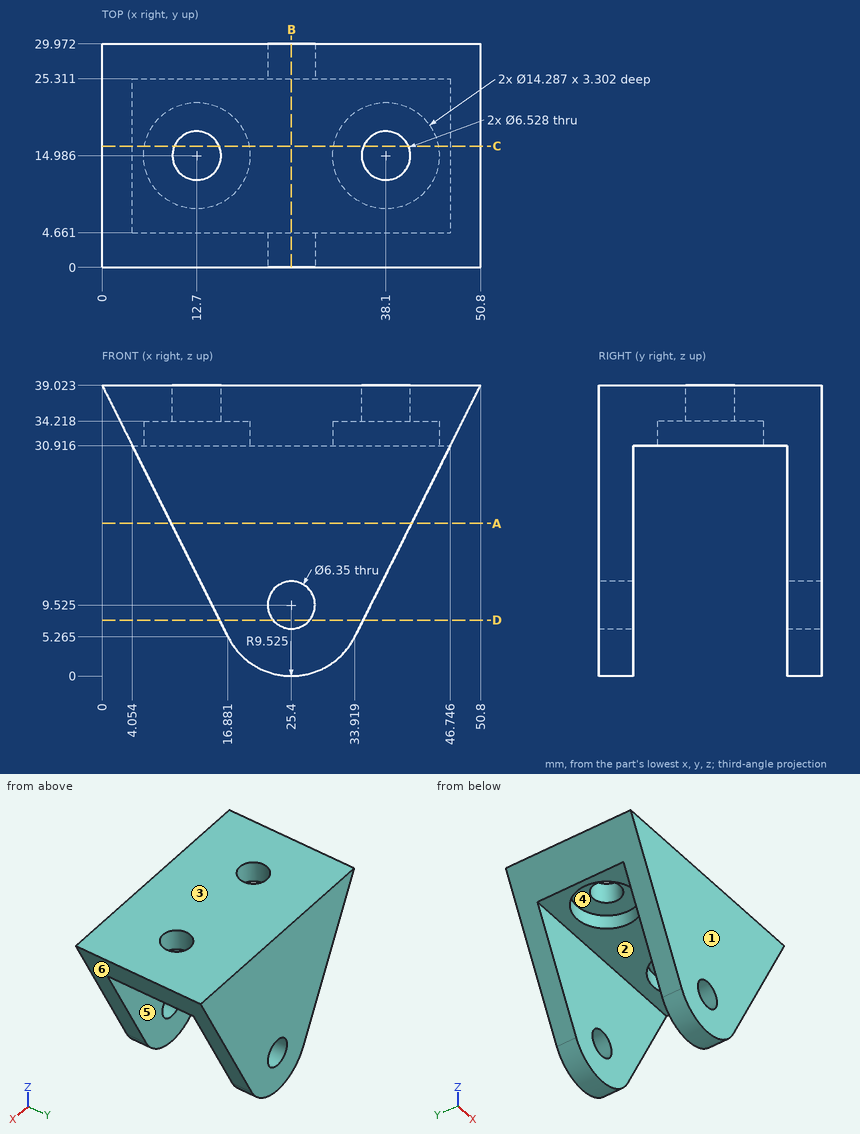
Geometry: see drawing. Coordinates: mm, zero at the bounding-box minimum. A direction names the side the tool comes from. Round coordinates to 2 decimals unless told otherwise and drop trailing zeros. Order: outer loops, then holes, each group sorted by start corner. A loop starts at its lowest first (then second) coordinate and runs counter-clockwise, first axis right, second up. Notation, with made-up numbers: (43.25, 2.25) - (64.25, 2.25) arc R35 ccw to (64.25, 38.25) - close; hole circle Ø3 at (64.5, 38.25). An arc over 180 degrees is marked (long way). Use a Markdown table: item, result. Add a question column.
1. Section query A-A (z = 20.5). Return the cut outline in (x, y).
2. Section query D-D (z = 7.5). Return the cut outline in (x, y) (1 decimal), then the cut area to 3 significant figures.
3. Set-up query: the marked faces 4, 5 and 6. Return all of +Z, -Z, +X, -X, +Y, -Y with unobstructed straight access to the full face (end or side cutting, diameter ignored); none if empty.
4. Section query C-C (y = 16.25). Return the cut outline in (x, z), then the cut area to 3 significant figures.
5. Line query: probe 1 along Y at (x, z) = (44.5, 27.5); probe 2 along X at (y, z) = (14.5, 36); probe 3 along Y at (x, z) = (12.7, 32.9). Output: solid intervals per line, ascending.
6. First-contact query: pin 1 (12 mm diameter, centred on y = 6, z = 17, fed in from -X); pin 2 (6 mm diameter, centred on y = 4.5, z = 12.5, fed in from -X); pin 3 (8 mm diameter, centred on x = 39.5, y = 9.5, fed in from -Z). Flat tips, straight axial feed; report the tip coordinate or a pass-through.
7. Mould query, pull axis Y, two halves, no side actions, for the marked faces 1, 2 and 3. Classes: +Y half, -Y half, draft (parallel to the pull), parting line (faces both ways), or undercut.
8. Section query B-B (x = 25.4). Return the cut outline in (y, z).
Derived:
| question | item | result |
|---|---|---|
| 1 | outline | (9.26, 0) - (41.54, 0) - (41.54, 4.66) - (9.26, 4.66) - close; (9.26, 25.31) - (41.54, 25.31) - (41.54, 29.97) - (9.26, 29.97) - close |
| 2 | outline | (15.8, 0) - (23, 0) - (23, 4.7) - (15.8, 4.7) - close; (15.8, 25.3) - (23, 25.3) - (23, 30) - (15.8, 30) - close; (27.8, 0) - (35, 0) - (35, 4.7) - (27.8, 4.7) - close; (27.8, 25.3) - (35, 25.3) - (35, 30) - (27.8, 30) - close |
| 2 | area | 134 mm2 |
| 3 | face 4 | -Z |
| 3 | face 5 | -Z, +X, -X |
| 3 | face 6 | -Z, +X, +Y, -Y |
| 4 | outline | (0, 39.02) - (4.05, 30.92) - (5.67, 30.92) - (5.67, 34.22) - (9.69, 34.22) - (9.69, 39.02) - close; (15.71, 34.22) - (19.73, 34.22) - (19.73, 30.92) - (31.07, 30.92) - (31.07, 34.22) - (35.09, 34.22) - (35.09, 39.02) - (15.71, 39.02) - close; (41.11, 34.22) - (45.13, 34.22) - (45.13, 30.92) - (46.75, 30.92) - (50.8, 39.02) - (41.11, 39.02) - close |
| 4 | area | 228 mm2 |
| 5 | probe 1 | 0 to 4.66, 25.31 to 29.97 |
| 5 | probe 2 | 1.51 to 9.47, 15.93 to 34.87, 41.33 to 49.29 |
| 5 | probe 3 | 0 to 7.84, 22.13 to 29.97 |
| 6 | pin 1 | x = 8.09 |
| 6 | pin 2 | x = 11.76 |
| 6 | pin 3 | z = 30.92 |
| 7 | face 1 | -Y half |
| 7 | face 2 | undercut |
| 7 | face 3 | draft |
| 8 | outline | (0, 0) - (4.66, 0) - (4.66, 6.35) - (0, 6.35) - close; (0, 12.7) - (4.66, 12.7) - (4.66, 30.92) - (25.31, 30.92) - (25.31, 12.7) - (29.97, 12.7) - (29.97, 39.02) - (0, 39.02) - close; (25.31, 0) - (29.97, 0) - (29.97, 6.35) - (25.31, 6.35) - close |
